from build123d import *

# Parameters (mm, degrees)
SKETCH2_W           = 23.2
SKETCH2_H           = 12.5
BOSS_EXTRUDE1_DEPTH = 16.4
SKETCH3_W           = 32.6
SKETCH3_H           = 12.5
SKETCH3_R           = 1
BOSS_EXTRUDE2_DEPTH = 2.4
SKETCH4_W           = 23.2
SKETCH4_H           = 12.5
BOSS_EXTRUDE3_DEPTH = 4.2
SKETCH5_R           = 6.25
SKETCH5_R_2         = 2.5
BOSS_EXTRUDE4_DEPTH = 4.3
SKETCH6_R           = 2.400000026
BOSS_EXTRUDE5_DEPTH = 3
SKETCH7_R           = 0.5
BOSS_EXTRUDE8_DEPTH = 2.54


with BuildPart() as part:
    # Sketch2 → Boss-Extrude1 (new body)
    with BuildSketch(Plane(origin=(0, 0, 0), x_dir=(1, 0, 0), z_dir=(0, 1, 0))):
        with Locations((11.6, 6.25)):
            Rectangle(SKETCH2_W, SKETCH2_H)
    extrude(amount=BOSS_EXTRUDE1_DEPTH)

    # Sketch3 → Boss-Extrude2 (add)
    with BuildSketch(Plane(origin=(0, 16.4, 0), x_dir=(1, 0, 0), z_dir=(0, 1, 0))):
        with Locations((11.6, 6.25)):
            Rectangle(SKETCH3_W, SKETCH3_H)
        with Locations(Location((-1.9, 6.25, 0), (0, 0, 270))):
            Circle(SKETCH3_R, mode=Mode.SUBTRACT)
        with Locations(Location((25.1, 6.25, 0), (0, 0, 270))):
            Circle(SKETCH3_R, mode=Mode.SUBTRACT)
    extrude(amount=BOSS_EXTRUDE2_DEPTH)

    # Sketch4 → Boss-Extrude3 (add)
    with BuildSketch(Plane(origin=(0, 18.8, 0), x_dir=(1, 0, 0), z_dir=(0, 1, 0))):
        with Locations((11.6, 6.25)):
            Rectangle(SKETCH4_W, SKETCH4_H)
    extrude(amount=BOSS_EXTRUDE3_DEPTH)

    # Sketch5 → Boss-Extrude4 (add)
    with BuildSketch(Plane(origin=(0, 23, 0), x_dir=(1, 0, 0), z_dir=(0, 1, 0))):
        with Locations((6.25, 6.25)):
            Circle(SKETCH5_R)
        with Locations((12.5, 6.25)):
            Circle(SKETCH5_R_2)
    extrude(amount=BOSS_EXTRUDE4_DEPTH)

    # Sketch6 → Boss-Extrude5 (add)
    with BuildSketch(Plane(origin=(0, 27.3, 0), x_dir=(1, 0, 0), z_dir=(0, 1, 0))):
        with Locations(Location((6.25, 6.25, 0), (0, 0, 270))):
            Circle(SKETCH6_R)
    extrude(amount=BOSS_EXTRUDE5_DEPTH)

    # Sketch7 → Boss-Extrude8 (add)
    with BuildSketch(Plane.ZY):
        with Locations(Location((-6.25, 5, 0), (0, 0, 180))):
            Circle(SKETCH7_R)
        with Locations(Location((-7.266, 5, 0), (0, 0, 180))):
            Circle(SKETCH7_R)
        with Locations(Location((-5.234, 5, 0), (0, 0, 180))):
            Circle(SKETCH7_R)
    extrude(amount=BOSS_EXTRUDE8_DEPTH)


solid = part.part
The listing builds one solid part. Answer for the finished solid, in the listing's coordinates (mm). A direction names the side the tool comes from. Coordinates: 2 decimals unless noted, no trailing zeros. Order: outer loops, then holes, each group sorted by start corner. A loop starts at its lowest first (then second) coordinate and runs counter-clockwise, first axis right, second up. Notation, with made-up numbers: (33.25, -38.5) -> (91.25, -38.5) arc R17 cw to (91.25, -12.5) -> close; hole circle Ø10 at (21.5, 88). An arc over 180 degrees is marked (long way). Answer in a Markdown table with one row per item. Add a question column.
Item 1: Each of these flat-tipped pins is pushed along its axis until it touches: P1, Ø0.5, axis at y = 5, z = -5.5, coming from the -X side; P2, Ø4, axis at y = 6, z = -3, coming from the +X side; P3, Ø1.3, axis at y = 20, z = -4.5, coming from the -X side. Where does it stop, or does it pass through?
Item 2: Find section C-C (y = 17). Write down the section's boundary in (x, z).
Item 3: Find section B-B (x = 24.5). Write down the section's boundary in (y, z).
Item 4: Which of the six approach directions +Z, -Z, +X, -X, +Y, -Y give full straight-line access (tool end or side, diameter ignored) to faces 1 (the face through (-3.4, 18.8, -6.3)), 2 (the face through (23.2, 8, -6)), 3 (the face through (-2.54, 5, -5)), 4 (the face through (0.005, 25.12, -6.49)), 5 (the face through (1, 23, -11))?
Item 5: Find the intervals of material crossed by L1, parallel to X at y = 17.45, z = -6.25; L2, parallel to Y at x = 10, z = -1.75; L3, parallel to Y at x = 21.5, z = -7.25, in increasing order. Write a range as from..to.
Item 6: Determine the mould class of faces 6 (the face through (1, 23, -2)), 7 (the face through (-1.224, 17.583, -6.987)), 8 (the face through (23.2, 21, -6)) for opening direction X: +X half, -X half, draft (parallel to the pull), parting line (faces both ways), or undercut.
Item 7: Find section D-D (x = 12.5). Write down the section's boundary in (y, z).
Item 8: Find section A-A (x = -1.9). Write down the section's boundary in (y, z).
Result set:
| question | item | result |
|---|---|---|
| 1 | P1 | stops at x = -2.54 |
| 1 | P2 | stops at x = 23.2 |
| 1 | P3 | stops at x = 0 |
| 2 | outline | (-4.7, -12.5) -> (27.9, -12.5) -> (27.9, 0) -> (-4.7, 0) -> close; hole circle Ø2 at (-1.9, -6.25); hole circle Ø2 at (25.1, -6.25) |
| 3 | outline | (16.4, -12.5) -> (18.8, -12.5) -> (18.8, -7.05) -> (16.4, -7.05) -> close; (16.4, -5.45) -> (18.8, -5.45) -> (18.8, 0) -> (16.4, 0) -> close |
| 4 | face 1 | +Z, -Z, -X, +Y |
| 4 | face 2 | +Z, -Z, +X, -Y |
| 4 | face 3 | +Z, -Z, -X, -Y |
| 4 | face 4 | +Y |
| 4 | face 5 | -Z, -X, +Y |
| 5 | L1 | x = -4.7..-2.9, -0.9..24.1, 26.1..27.9 |
| 5 | L2 | y = 0..27.3 |
| 5 | L3 | y = 0..23 |
| 6 | face 6 | draft |
| 6 | face 7 | undercut |
| 6 | face 8 | +X half |
| 7 | outline | (0, -12.5) -> (23, -12.5) -> (23, -8.75) -> (27.3, -8.75) -> (27.3, -3.75) -> (23, -3.75) -> (23, 0) -> (0, 0) -> close |
| 8 | outline | circle Ø1 at (5, -7.27); circle Ø1 at (5, -6.25); circle Ø1 at (5, -5.23); (16.4, -12.5) -> (18.8, -12.5) -> (18.8, -7.25) -> (16.4, -7.25) -> close; (16.4, -5.25) -> (18.8, -5.25) -> (18.8, 0) -> (16.4, 0) -> close |
